The listing builds one solid part. Answer for the finished solid, in the listing's coordinates (mm). Face numbers are marked on the shaded views. A direction names the side the tool comes from. Coordinates: 2 decimals unless noted, no trailing zeros. Order: outer loops, then holes, each group sorted by start corner. A loop starts at its lowest first (then second) coordinate and runs counter-clockwise, first axis right, second up. Notation, with made-up numbers: (-27.5, -7) -> (6.5, -7) arc R21 cw to (6.5, 31) -> close; hole circle Ø6 at (-13, 50). An arc over 180 degrees is marked (long way). Return JSON: item names as keys, results as strings.
from build123d import *

# Parameters (mm, degrees)
F0_R          = 7
F1_DEPTH      = 38
F3_DEPTH      = 57
F4_DEPTH      = 54
F5_W          = 121
F5_H          = 16
F6_DEPTH      = 57
F7_DEPTH      = 54
F7_DEPTH_BACK = 38


with BuildPart() as f1:
    # F0 (on Front) → F1 (new body)
    with BuildSketch(Plane.XZ):
        Polygon((0, 46), (0, 0), (22, 0), (22, 28.847458), align=None)
        Polygon((22, 28.847458), (22, 0), (59, 0), align=None)
        Polygon((121, 57), (62, 57), (121, 11), align=None)
        Polygon((0, 57), (0, 46), (22, 28.847458), (59, 0), (121, 0), (121, 11), (62, 57), align=None)
        with Locations((77, 12)):
            Circle(F0_R, mode=Mode.SUBTRACT)
        with Locations((44, 41)):
            Circle(F0_R, mode=Mode.SUBTRACT)
    extrude(amount=-F1_DEPTH)

    # F2 (on face) → F3 (cut)
    with BuildSketch(Plane(origin=(0, 0, 0), x_dir=(1, 0, 0), z_dir=(0, 0, -1))):
        Polygon((121, 0), (22, 0), (121, -32), align=None)
    extrude(amount=-F3_DEPTH, mode=Mode.SUBTRACT)

    # F0 (on Front) → F4 (cut)
    with BuildSketch(Plane.XZ):
        Polygon((0, 57), (0, 46), (22, 28.847458), (59, 0), (121, 0), (121, 11), (62, 57), align=None)
        with Locations((77, 12)):
            Circle(F0_R, mode=Mode.SUBTRACT)
        with Locations((44, 41)):
            Circle(F0_R, mode=Mode.SUBTRACT)
    extrude(amount=-F4_DEPTH, mode=Mode.SUBTRACT)

    # F5 (on Top) → F6 (join)
    with BuildSketch(Plane.XY):
        with Locations((60.5, 46)):
            Rectangle(F5_W, F5_H)
    extrude(amount=F6_DEPTH)

    # F0 (on Front) → F7 (cut, two sides)
    with BuildSketch(Plane.XZ) as f7_sk:
        with Locations((44, 41)):
            Circle(F0_R)
        with Locations((77, 12)):
            Circle(F0_R)
    extrude(amount=-F7_DEPTH, mode=Mode.SUBTRACT)
    extrude(f7_sk.sketch, amount=-F7_DEPTH_BACK, mode=Mode.SUBTRACT)


solid = f1.part
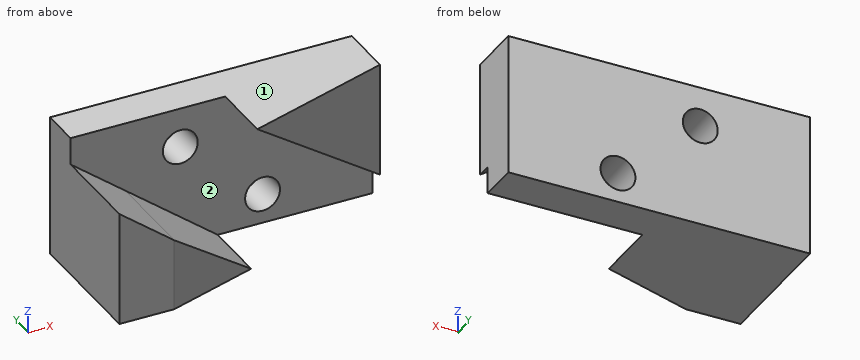
1. The part is cut by section A-A on y = 41. Give the vertices of the cut face in (x, z).
Answer block:
{"outline": "(0, 0) -> (121, 0) -> (121, 57) -> (0, 57) -> close; hole circle Ø14 at (44, 41); hole circle Ø14 at (77, 12)"}
2. Consider line 1 (Z direction, x = 44, y = 50); line 2 (Y direction, x = 111, z = 11); line 3 (Z direction, x = 77, y = 48). Determine where each line is inside the solid, lowest interval first. Write a range as from..to.
Answer block:
{"line 1": "z = 0..34, 48..57", "line 2": "y = 38..54", "line 3": "z = 0..5, 19..57"}
3. For the marked faces 1 and 2, determine the directions among +Z, -Z, +X, -X, +Y, -Y from which every point of the face is accessible in a straight line to the end or side of a thin tool.
Answer block:
{"face 1": "+Z, +X, -X, +Y, -Y", "face 2": "-Y"}
4. The part is cut by section B-B on z = 41. Give the vertices of the cut face in (x, y).
Answer block:
{"outline": "(0, 0) -> (6.41, 0) -> (6.41, 38) -> (37, 38) -> (37, 54) -> (0, 54) -> close; (51, 38) -> (82.52, 38) -> (82.52, 19.56) -> (121, 32) -> (121, 54) -> (51, 54) -> close"}
5. The part is cut by section D-D on y = 29. Give the vertices of the cut face in (x, z).
Answer block:
{"outline": "(0, 0) -> (59, 0) -> (0, 46) -> close; (62, 57) -> (111.72, 18.24) -> (111.72, 57) -> close"}
6. Each of these flat-tipped pins is pushed along its axis until it touches: pin 1 Ø8 at (y, z) = (7, 49) entering from -X; pin 2 Ø1 at (x, z) = (91, 29.5) entering from -Y; pin 3 Ø11 at (x, z) = (44, 41) entering from -Y; pin 4 Ø2 at (x, z) = (91.5, 46) entering from -Y. Where does it stop, or does it pass through?
Answer block:
{"pin 1": "stops at x = 0", "pin 2": "stops at y = 38", "pin 3": "passes through", "pin 4": "stops at y = 22.14"}
7. The part is cut by section C-C on x = 45. Give the vertices of the cut face in (y, z), and give its area (3 significant figures).
Answer block:
{"outline": "(7.43, 0) -> (54, 0) -> (54, 34.07) -> (38, 34.07) -> (38, 10.92) -> (7.43, 10.92) -> close; (38, 47.93) -> (54, 47.93) -> (54, 57) -> (38, 57) -> close", "area": "1,020 mm2"}
